Geometry: see drawing. Coordinates: mm, zero at the bounding-box minimum. Coordinates: 2 decimals unless noted, no trailing zeros. Loops run counter-clockwise (first coordinate to the right, second up) from the corner with the lowest first, then second, coordinate; pieces in that order, holes last. Notation, with made-up numbers: M 24,52.5 L 72,52.5 A17 cw 72,80.5 Z; hole C 81.5,42 d9. An arc over 180 degrees is marked long. One line per question, with ' | ' between items. Start each with the question number.
1. Section query D-D, the plane x = 39.5. Output: boundary loops of the cut face in (y, z).
2. Section query C-C, the plane z = 0.6. State how many separate pieces and enclosed holes the cut face has, and give its area (3 significant figures).
3. Section query A-A, the plane x = 97. Output: boundary loops of the cut face in (y, z), and give its area (3 significant figures).
4. Pin query (flat end, axial travel): P1, Ø0.6, axis at x = 96, z = 1.5, coming from the -Y side; P2, Ø0.6, axis at y = 47.5, z = 1.5, coming from the +X side; P3, Ø3, axis at x = 41, y = 48.5, coming from the -Z side; P4, Ø1, axis at x = 92, z = 0.5, coming from the +Y side. Return the tip coordinate at first contact, or that it passes through.
5. Section query B-B, the plane y = 33. Output: boundary loops of the cut face in (x, z), and give its area (3 significant figures).
6. Ray query, probe 1 along X at (y, z) = (39.5, 0.5); probe 2 along Y at (x, z) = (146.5, 1.8); probe 3 along Y at (x, z) = (101.5, 0.7). Return the intervals inside material, ascending.
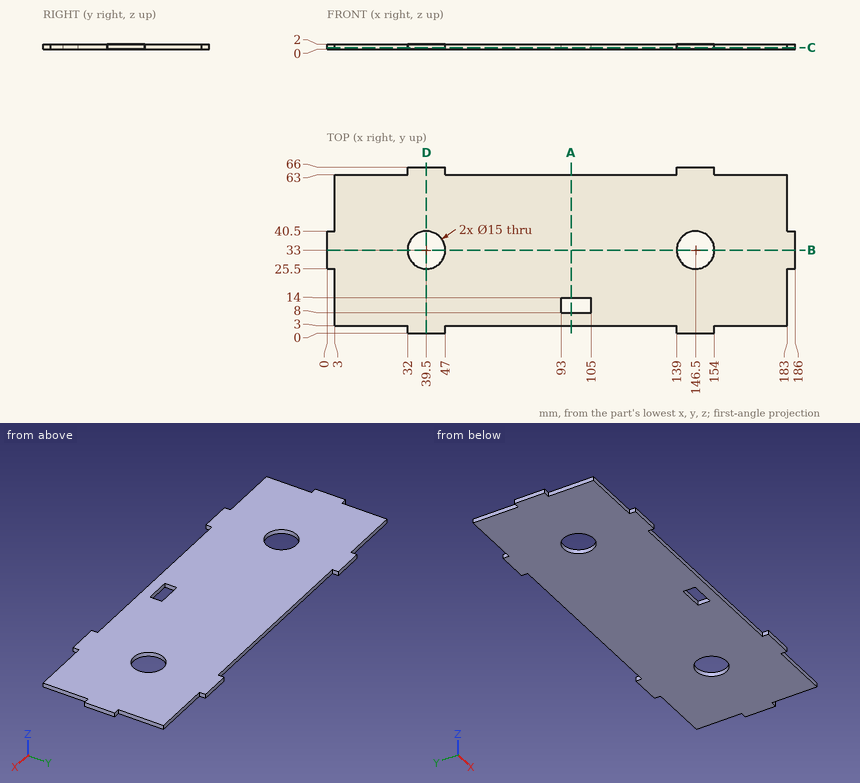
Taken from the geometry:
1) outline: M 0,0 L 25.5,0 L 25.5,2 L 0,2 Z; M 40.5,0 L 66,0 L 66,2 L 40.5,2 Z
2) separate pieces: 1 | enclosed holes: 3 | area: 10,600 mm^2
3) outline: M 3,0 L 8,0 L 8,2 L 3,2 Z; M 14,0 L 63,0 L 63,2 L 14,2 Z | area: 108 mm^2
4) P1: y = 3 | P2: x = 183 | P3: z = 0 | P4: y = 63
5) outline: M 0,0 L 32,0 L 32,2 L 0,2 Z; M 47,0 L 139,0 L 139,2 L 47,2 Z; M 154,0 L 186,0 L 186,2 L 154,2 Z | area: 312 mm^2
6) probe 1: 0 to 35.76, 43.24 to 142.76, 150.24 to 186 | probe 2: 0 to 25.5, 40.5 to 66 | probe 3: 3 to 8, 14 to 63
